Read the model definition and answer for the solid it produces. Units are mm, in the model's axes. Face numbers are marked on the shaded views. Coordinates: 2 decimals unless noted, no trailing zeros. Order: outer loops, then holes, each group sorted by start corner. A loop starts at its lowest first (then second) coordinate and runs counter-clockwise, first axis right, second up. Notation, with made-up numbers: M 46.5,62.25 L 95.5,62.25 A17 cw 95.5,81.25 Z; hole C 75,55 d7. An arc over 180 degrees is marked long. Use a Markdown table: item, result. Add a question column.
1) Each of these flat-tipped pins is pushed along its axis until it touches: pin 1 Ø1 at (y, z) = (-6, 4) entering from -X; pin 2 Ø1 at (x, z) = (8, 1.5) entering from -Y; pin 3 Ø4 at (y, z) = (-3, 1) entering from -X. Where does it stop, or does it pass through?
2) Find section C-C on x = -3.5. Write down the section's boundary in (y, z).
3) The mould has two halves that part along Y. Classify the marked faces 1, 2 and 3: released by +Y, released by -Y, zero draft, split by the parting line, or undercut.
4) Find the intervals of material crossed by probe 1 along Y at (x, z) = (0, 3.5); probe 2 along X at (y, z) = (3, 1); probe 3 along Y at (x, z) = (2.75, 4.75), in increasing order. Write a range as [from, to].
5) Find section B-B on z = 2.5. Write down the section's boundary in (x, y), plus the area to 3 significant figures.
6) Find section A-A on x = 0. Write down the section's boundary in (y, z).
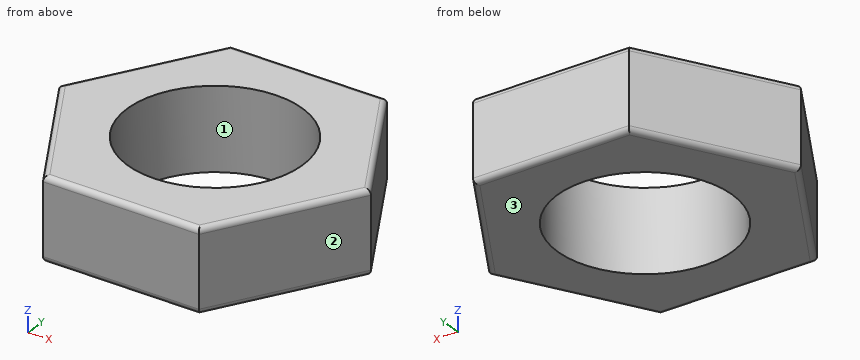
from build123d import *

# Parameters (mm, degrees)
EXTRUDE_1_DEPTH     = 7.5
SKETCH_3_R          = 8
CUT_EXTRUDE_1_DEPTH = 21.514222708
FILLET_1_R          = 0.5


with BuildPart() as part:
    # 草图2 → 凸台-拉伸1 (new body)
    with BuildSketch(Plane.XY):
        Polygon((7.216878365, -12.5), (14.43375673, 0), (7.216878365, 12.5), (-7.216878365, 12.5), (-14.43375673, 0), (-7.216878365, -12.5), align=None)
    extrude(amount=EXTRUDE_1_DEPTH)

    # 草图3 → 切除-拉伸1 (cut, through all)
    with BuildSketch(Plane.XY.offset(7.5)):
        Circle(SKETCH_3_R)
    extrude(amount=-CUT_EXTRUDE_1_DEPTH, mode=Mode.SUBTRACT)

    # 圆角1
    fillet_1_edges = [part.edges().sort_by_distance(p)[0] for p in [
        (10.825317547, 6.25, 7.5),
        (0, 12.5, 7.5),
        (-10.825317547, 6.25, 7.5),
        (-10.825317547, -6.25, 7.5),
        (0, -12.5, 7.5),
        (-10.825317547, -6.25, 0),
        (-10.825317547, 6.25, 0),
        (0, 12.5, 0),
        (10.825317547, -6.25, 7.5),
        (10.825317547, 6.25, 0),
        (10.825317547, -6.25, 0),
        (0, -12.5, 0),
    ]]
    fillet(fillet_1_edges, radius=FILLET_1_R)


solid = part.part
Check result:
| question | item | result |
|---|---|---|
| 1 | pin 1 | stops at x = -11.26 |
| 1 | pin 2 | stops at y = -12.01 |
| 1 | pin 3 | stops at x = -13.86 |
| 2 | outline | M -12.5,0.5 A0.5 ccw -12,0 L -7.19,0 L -7.19,7.5 L -12,7.5 A0.5 ccw -12.5,7 Z; M 7.19,0 L 12,0 A0.5 ccw 12.5,0.5 L 12.5,7 A0.5 ccw 12,7.5 L 7.19,7.5 Z |
| 3 | face 1 | undercut |
| 3 | face 2 | released by -Y |
| 3 | face 3 | zero draft |
| 4 | probe 1 | y = [-12.5, -8], [8, 12.5] |
| 4 | probe 2 | x = [-12.7, -7.42], [7.42, 12.7] |
| 4 | probe 3 | y = [-12.5, -7.51], [7.51, 12.5] |
| 5 | outline | M -14.43,0 L -7.22,-12.5 L 7.22,-12.5 L 14.43,0 L 7.22,12.5 L -7.22,12.5 Z; hole C 0,0 d16 |
| 5 | area | 340 mm2 |
| 6 | outline | M -12.5,0.5 A0.5 ccw -12,0 L -8,0 L -8,7.5 L -12,7.5 A0.5 ccw -12.5,7 Z; M 8,0 L 12,0 A0.5 ccw 12.5,0.5 L 12.5,7 A0.5 ccw 12,7.5 L 8,7.5 Z |
